```python
from build123d import *

# Parameters (mm, degrees)
SKETCH_1_W          = 150
SKETCH_1_H          = 38
EXTRUDE_1_DEPTH     = 3
CUT_EXTRUDE_1_REACH = 79.427
SKETCH_2_R          = 2.5
CUT_EXTRUDE_2_REACH = 79.427
SKETCH_4_R          = 2.5


with BuildPart() as part:
    # Sketch 1 → Extrude 1 (new body)
    with BuildSketch(Plane.XY):
        Rectangle(SKETCH_1_W, SKETCH_1_H)
    extrude(amount=EXTRUDE_1_DEPTH)

    # Sketch 2 → Cut-Extrude 1 (cut, up to next)
    with BuildSketch(Plane(origin=(0, 0, 0), x_dir=(-1, 0, 0), z_dir=(0, 0, -1)), mode=Mode.PRIVATE) as cut_extrude_1_sk1:
        with Locations((-61, 0)):
            Circle(SKETCH_2_R)
    cut_extrude_1_tool1 = extrude(cut_extrude_1_sk1.sketch, amount=-CUT_EXTRUDE_1_REACH, mode=Mode.PRIVATE) & part.part
    # Sketch 2 → Cut-Extrude 1 (cut, up to next)
    with BuildSketch(Plane(origin=(0, 0, 0), x_dir=(-1, 0, 0), z_dir=(0, 0, -1)), mode=Mode.PRIVATE) as cut_extrude_1_sk2:
        with Locations((-43, 0)):
            Circle(SKETCH_2_R)
    cut_extrude_1_tool2 = extrude(cut_extrude_1_sk2.sketch, amount=-CUT_EXTRUDE_1_REACH, mode=Mode.PRIVATE) & part.part
    cut_extrude_1_1 = cut_extrude_1_tool1.solids().sort_by_distance((61, 0, 0))[0]
    add(cut_extrude_1_1, mode=Mode.SUBTRACT)
    cut_extrude_1_2 = cut_extrude_1_tool2.solids().sort_by_distance((43, 0, 0))[0]
    add(cut_extrude_1_2, mode=Mode.SUBTRACT)
    cut_extrude_1 = cut_extrude_1_1 + cut_extrude_1_2  # Cut-Extrude 1 as one shape, for the pattern or mirror that repeats it

    # Mirror 1: Cut-Extrude 1 across plane
    add(cut_extrude_1.mirror(Plane(origin=(0, 0, 0), x_dir=(0, 0, 1), z_dir=(1, 0, 0))), mode=Mode.SUBTRACT)

    # Sketch 4 → Cut-Extrude 2 (cut, up to next)
    with BuildSketch(Plane(origin=(0, 0, 0), x_dir=(-1, 0, 0), z_dir=(0, 0, -1)), mode=Mode.PRIVATE) as cut_extrude_2_sk1:
        with Locations((0, -6)):
            Circle(SKETCH_4_R)
    cut_extrude_2_tool1 = extrude(cut_extrude_2_sk1.sketch, amount=-CUT_EXTRUDE_2_REACH, mode=Mode.PRIVATE) & part.part
    # Sketch 4 → Cut-Extrude 2 (cut, up to next)
    with BuildSketch(Plane(origin=(0, 0, 0), x_dir=(-1, 0, 0), z_dir=(0, 0, -1)), mode=Mode.PRIVATE) as cut_extrude_2_sk2:
        with Locations((0, 12)):
            Circle(SKETCH_4_R)
    cut_extrude_2_tool2 = extrude(cut_extrude_2_sk2.sketch, amount=-CUT_EXTRUDE_2_REACH, mode=Mode.PRIVATE) & part.part
    add(cut_extrude_2_tool1.solids().sort_by_distance((0, -6, 0))[0], mode=Mode.SUBTRACT)
    add(cut_extrude_2_tool2.solids().sort_by_distance((0, 12, 0))[0], mode=Mode.SUBTRACT)


solid = part.part
```
Here's how the part is built. I have some questions about the finished solid (model axes, mm). Coordinates: 2 decimals unless noted, no trailing zeros. Order: outer loops, then holes, each group sorted by start corner. A loop starts at its lowest first (then second) coordinate and runs counter-clockwise, first axis right, second up. Notation, with made-up numbers: M 6.25,-3 L 26.25,-3 A29 ccw 26.25,31 Z; hole C 84,63 d6. An arc over 180 degrees is marked long. Answer as a JSON object with one key per item and string values. Group by question number.
(1) Suppose I cut it at D-D, the plane z = 0.5. Please give me the cut outline in (x, y).
(2) Suppose I cut it at C-C, the plane x = 61. Please give me the cut outline in (y, z).
(3) Suppose I cut it at A-A, the plane y = 12. Please give me the cut outline in (x, z), then the cut area to 3 significant figures.
(4) Suppose I cut it at B-B, the plane x = 0. Please give me the cut outline in (y, z).
(5) For pin 1 (8 mm diameter, centred on x = 0, y = 12, fed in from -Z); pin 2 (4.5 mm diameter, centred on x = 0, y = -6, fed in from -Z), each with a flat end and sliding along its axis, tell me the tip position at first contact or that it passes through.
(6) I need wall thicknesses on probe 1 along Y at (x, z) = (-61, 1.85); probe 2 along X at (y, z) = (2, 0.55); probe 3 along Y at (x, z) = (-42, 1.7). Which ranges of each line are inside material? Lowest first, please.
(7) If we mould it in two halves opening along X, with no side actions, what happens to faces 1 (the face through (-1, 0, 0)), 2 (the face through (-75, 0, 1)), 3 (the face through (0.33, -3.52, 1.48))? For each: released by +X, released by -X, zero draft, split by the parting line, or undercut.
Values found:
{
 "1": {"outline": "M -75,-19 L 75,-19 L 75,19 L -75,19 Z; hole C -61,0 d5; hole C -43,0 d5; hole C 0,-6 d5; hole C 0,12 d5; hole C 43,0 d5; hole C 61,0 d5"},
 "2": {"outline": "M -19,0 L -2.5,0 L -2.5,3 L -19,3 Z; M 2.5,0 L 19,0 L 19,3 L 2.5,3 Z"},
 "3": {"outline": "M -75,0 L -2.5,0 L -2.5,3 L -75,3 Z; M 2.5,0 L 75,0 L 75,3 L 2.5,3 Z", "area": "435 mm^2"},
 "4": {"outline": "M -19,0 L -8.5,0 L -8.5,3 L -19,3 Z; M -3.5,0 L 9.5,0 L 9.5,3 L -3.5,3 Z; M 14.5,0 L 19,0 L 19,3 L 14.5,3 Z"},
 "5": {"pin 1": "stops at z = 0", "pin 2": "passes through"},
 "6": {"probe 1": "y = -19 to -2.5, 2.5 to 19", "probe 2": "x = -75 to -62.5, -59.5 to -44.5, -41.5 to 41.5, 44.5 to 59.5, 62.5 to 75", "probe 3": "y = -19 to -2.29, 2.29 to 19"},
 "7": {"face 1": "zero draft", "face 2": "released by -X", "face 3": "undercut"}
}
